Check sheet for the modelled part. Datum: model origin and axes. Units: mm. Round coordinates to 2 decimals unless told otherwise and drop trailing zeros. Loops run counter-clockwise (first coordinate to the right, second up) from the corner with the lowest first, then second, coordinate; pieces in that order, holes last. Notation, with made-up numbers: (69, -13) - (106, -13) arc R9 cw to (106, 2) - close; hole circle Ø9 at (88.25, 33). An arc over 180 degrees is marked (long way). Return JSON: item names as keys, results as strings.
from build123d import *

# Parameters (mm, degrees)
F0_W     = 150
F0_H     = 6
F1_DEPTH = 40
F3_DEPTH = 40.001


with BuildPart() as f1:
    # F0 (on Front) → F1 (new body)
    with BuildSketch(Plane.XZ):
        with Locations((75, 3)):
            Rectangle(F0_W, F0_H)
    extrude(amount=-F1_DEPTH)

    # F2 (on face) → F3 (cut, through all)
    with BuildSketch(Plane.XZ):
        with BuildLine():
            ThreePointArc((2.5, 6), (5, 3.5), (7.5, 6))
            Line((7.5, 6), (2.5, 6))
        make_face()
        with BuildLine():
            Line((17.5, 6), (12.5, 6))
            ThreePointArc((12.5, 6), (15, 3.5), (17.5, 6))
        make_face()
        with BuildLine():
            Line((27.5, 6), (22.5, 6))
            ThreePointArc((22.5, 6), (25, 3.5), (27.5, 6))
        make_face()
        with BuildLine():
            Line((37.5, 6), (32.5, 6))
            ThreePointArc((32.5, 6), (35, 3.5), (37.5, 6))
        make_face()
        with BuildLine():
            Line((142.5, 6), (147.5, 6))
            ThreePointArc((147.5, 6), (145, 8.5), (142.5, 6))
        make_face()
        with BuildLine():
            ThreePointArc((142.5, 6), (145, 3.5), (147.5, 6))
            Line((147.5, 6), (142.5, 6))
        make_face()
        with BuildLine():
            Line((47.5, 6), (42.5, 6))
            ThreePointArc((42.5, 6), (45, 3.5), (47.5, 6))
        make_face()
        with BuildLine():
            Line((132.5, 6), (137.5, 6))
            ThreePointArc((137.5, 6), (135, 8.5), (132.5, 6))
        make_face()
        with BuildLine():
            ThreePointArc((132.5, 6), (135, 3.5), (137.5, 6))
            Line((137.5, 6), (132.5, 6))
        make_face()
        with BuildLine():
            Line((57.5, 6), (52.5, 6))
            ThreePointArc((52.5, 6), (55, 3.5), (57.5, 6))
        make_face()
        with BuildLine():
            Line((122.5, 6), (127.5, 6))
            ThreePointArc((127.5, 6), (125, 8.5), (122.5, 6))
        make_face()
        with BuildLine():
            ThreePointArc((122.5, 6), (125, 3.5), (127.5, 6))
            Line((127.5, 6), (122.5, 6))
        make_face()
        with BuildLine():
            Line((67.5, 6), (62.5, 6))
            ThreePointArc((62.5, 6), (65, 3.5), (67.5, 6))
        make_face()
        with BuildLine():
            Line((112.5, 6), (117.5, 6))
            ThreePointArc((117.5, 6), (115, 8.5), (112.5, 6))
        make_face()
        with BuildLine():
            ThreePointArc((112.5, 6), (115, 3.5), (117.5, 6))
            Line((117.5, 6), (112.5, 6))
        make_face()
        with BuildLine():
            Line((77.5, 6), (72.5, 6))
            ThreePointArc((72.5, 6), (75, 3.5), (77.5, 6))
        make_face()
        with BuildLine():
            ThreePointArc((102.5, 6), (105, 3.5), (107.5, 6))
            Line((107.5, 6), (102.5, 6))
        make_face()
        with BuildLine():
            Line((87.5, 6), (82.5, 6))
            ThreePointArc((82.5, 6), (85, 3.5), (87.5, 6))
        make_face()
        with BuildLine():
            ThreePointArc((92.5, 6), (95, 3.5), (97.5, 6))
            Line((97.5, 6), (92.5, 6))
        make_face()
    extrude(amount=-F3_DEPTH, mode=Mode.SUBTRACT)


solid = f1.part
Q1. Scan lines: probe 1 along Z at (x, y) = (125, 31.5); probe 2 along Z at (x, y) = (87, 32). Record each from-to range of solid material in increasing order. Write a range as [from, to].
Answer key:
{"probe 1": "z = [0, 3.5]", "probe 2": "z = [0, 4.5]"}
Q2. Draft check along X on faces 1 (the face through (150, 20, 3)), 2 (the face through (134.9, 19.7, 3.5)), 3 (the face through (130, 20, 6)), 4 (the face through (0, 20, 3)). Enter one of: released by +X, released by -X, zero draft, split by the parting line, or undercut.
Answer key:
{"face 1": "released by +X", "face 2": "undercut", "face 3": "zero draft", "face 4": "released by -X"}
Q3. Sectioned sample at B-B (z = 4.85). State how many separate pieces and enclosed holes the cut face has, plus the area to 3 significant figures.
Answer key:
{"separate pieces": "16", "enclosed holes": "0", "area": "3,340 mm²"}
Q4. Sectioned sample at C-C (x = 45). Enter the section's corners in (y, z).
Answer key:
{"outline": "(0, 0) - (40, 0) - (40, 3.5) - (0, 3.5) - close"}
Q5. Depth check by flat-ended pin: P1, Ø2, axis at x = 74, y = 35.5, coming from the +Z side. Enter the tip coordinate at first touch or a pass-through.
Answer key:
{"P1": "stops at z = 4.5"}
